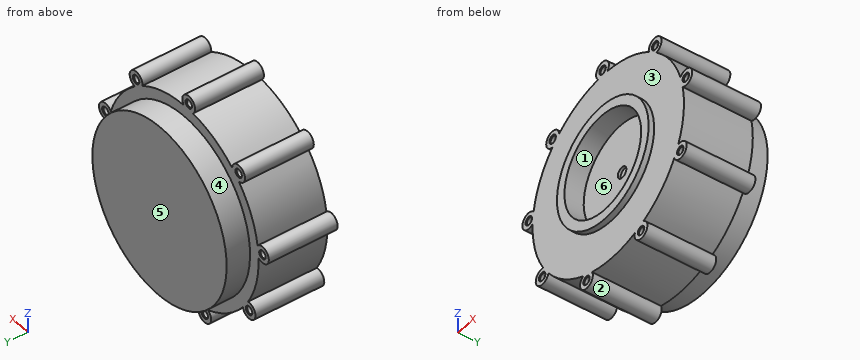
```python
from build123d import *

# Parameters (mm, degrees)
SKETCH_1_R                   = 3
SKETCH_1_R_2                 = 35.5
EXTRUDE_1_DEPTH              = 25
HOLE_WIZARD_M3_1_D           = 2.5
HOLE_WIZARD_M3_1_DEPTH       = 8
HOLE_WIZARD_M3_1_CSINK_D     = 3.05
HOLE_WIZARD_M3_1_CSINK_ANGLE = 90
HOLE_WIZARD_M3_1_TIP         = 0.751075774
SKETCH_7_R                   = 21.5
SKETCH_7_R_2                 = 18
EXTRUDE_3_DEPTH              = 2
CUT_EXTRUDE_START            = -5
SKETCH_8_R                   = 18
CUT_EXTRUDE_2_DEPTH          = 5
SKETCH_9_R                   = 2
CUT_EXTRUDE_3_DEPTH          = 1
SKETCH_11_R                  = 31.5
EXTRUDE_4_DEPTH              = 8.5
HOLE_WIZARD_M3_4_D           = 2.5
HOLE_WIZARD_M3_4_DEPTH       = 8
HOLE_WIZARD_M3_4_CSINK_D     = 3.05
HOLE_WIZARD_M3_4_CSINK_ANGLE = 90
HOLE_WIZARD_M3_4_TIP         = 0.751075774


with BuildPart() as part:
    # 草图1 → 凸台-拉伸1 (new body)
    with BuildSketch(Plane(origin=(0, 0, 0), x_dir=(1, 0, 0), z_dir=(0, 1, 0))):
        with Locations((-31.034181612, 21.050643022)):
            Circle(SKETCH_1_R)
        Circle(SKETCH_1_R_2)
        with Locations((-37.304654882, -3.822659306)):
            Circle(SKETCH_1_R)
        with Locations((-26.119865536, -26.907296861)):
            Circle(SKETCH_1_R)
        with Locations((-2.713300817, -37.401711173)):
            Circle(SKETCH_1_R)
        with Locations((21.96284751, -30.395449154)):
            Circle(SKETCH_1_R)
        with Locations((36.362335397, -9.166818668)):
            Circle(SKETCH_1_R)
        with Locations((33.747482429, 16.351068151)):
            Circle(SKETCH_1_R)
        with Locations((15.341807372, 34.21810846)):
            Circle(SKETCH_1_R)
        with Locations((-10.24246986, 36.074115528)):
            Circle(SKETCH_1_R)
        Circle(SKETCH_1_R_2)
        with Locations((-37.304654882, -3.822659306)):
            Circle(SKETCH_1_R)
        Circle(SKETCH_1_R_2)
        with Locations((-37.304654882, -3.822659306)):
            Circle(SKETCH_1_R)
        Circle(SKETCH_1_R_2)
        with Locations((-26.119865536, -26.907296861)):
            Circle(SKETCH_1_R)
        Circle(SKETCH_1_R_2)
        with Locations((-26.119865536, -26.907296861)):
            Circle(SKETCH_1_R)
        Circle(SKETCH_1_R_2)
        with Locations((-2.713300817, -37.401711173)):
            Circle(SKETCH_1_R)
        Circle(SKETCH_1_R_2)
        with Locations((-2.713300817, -37.401711173)):
            Circle(SKETCH_1_R)
        Circle(SKETCH_1_R_2)
        with Locations((21.96284751, -30.395449154)):
            Circle(SKETCH_1_R)
        Circle(SKETCH_1_R_2)
        with Locations((21.96284751, -30.395449154)):
            Circle(SKETCH_1_R)
        Circle(SKETCH_1_R_2)
        with Locations((36.362335397, -9.166818668)):
            Circle(SKETCH_1_R)
        Circle(SKETCH_1_R_2)
        with Locations((36.362335397, -9.166818668)):
            Circle(SKETCH_1_R)
        Circle(SKETCH_1_R_2)
        with Locations((33.747482429, 16.351068151)):
            Circle(SKETCH_1_R)
        Circle(SKETCH_1_R_2)
        with Locations((33.747482429, 16.351068151)):
            Circle(SKETCH_1_R)
        Circle(SKETCH_1_R_2)
        with Locations((15.341807372, 34.21810846)):
            Circle(SKETCH_1_R)
        Circle(SKETCH_1_R_2)
        with Locations((15.341807372, 34.21810846)):
            Circle(SKETCH_1_R)
        Circle(SKETCH_1_R_2)
        with Locations((-10.24246986, 36.074115528)):
            Circle(SKETCH_1_R)
        Circle(SKETCH_1_R_2)
        with Locations((-10.24246986, 36.074115528)):
            Circle(SKETCH_1_R)
        Circle(SKETCH_1_R_2)
        with Locations((-31.034181612, 21.050643022)):
            Circle(SKETCH_1_R)
        Circle(SKETCH_1_R_2)
        with Locations((-31.034181612, 21.050643022)):
            Circle(SKETCH_1_R)
    extrude(amount=EXTRUDE_1_DEPTH)

    # M3 螺纹孔1
    with Locations(Plane(origin=(-26.119865536, 0, 26.907296861), x_dir=(0, 0, -1), z_dir=(0, -1, 0))):
        with Locations((0, 0), (-10.494414312, 23.406564719), (-3.488152293, 48.082713046), (17.740478193, 62.482200933), (43.258365012, 59.867347965), (61.125405321, 41.461672908), (62.981412389, 15.877395676), (47.957939883, -4.914316076), (23.084637555, -11.184789346)):
            CounterSinkHole(HOLE_WIZARD_M3_1_D / 2, HOLE_WIZARD_M3_1_CSINK_D / 2, depth=HOLE_WIZARD_M3_1_DEPTH, counter_sink_angle=HOLE_WIZARD_M3_1_CSINK_ANGLE)
            with Locations((0, 0, -(HOLE_WIZARD_M3_1_DEPTH + HOLE_WIZARD_M3_1_TIP / 2))):  # 118° drill point
                Cone(0, HOLE_WIZARD_M3_1_D / 2, HOLE_WIZARD_M3_1_TIP, mode=Mode.SUBTRACT)

    # 草图7 → 凸台-拉伸3 (add)
    with BuildSketch(Plane.XZ):
        with Locations(Location((0, 0, 0), (0, 0, 90))):
            Circle(SKETCH_7_R)
        with Locations(Location((0, 0, 0), (0, 0, 270))):
            Circle(SKETCH_7_R_2, mode=Mode.SUBTRACT)
    extrude(amount=EXTRUDE_3_DEPTH)

    # 草图8 → 切除-拉伸2 (cut)
    with BuildSketch(Plane.XZ.offset(CUT_EXTRUDE_START)):
        with Locations(Location((0, 0, 0), (0, 0, 270))):
            Circle(SKETCH_8_R)
    extrude(amount=CUT_EXTRUDE_2_DEPTH, mode=Mode.SUBTRACT)

    # 草图9 → 切除-拉伸3 (cut)
    with BuildSketch(Plane.XZ.offset(-5)):
        with Locations(Location((0, 0, 0), (0, 0, 270))):
            Circle(SKETCH_9_R)
    extrude(amount=-CUT_EXTRUDE_3_DEPTH, mode=Mode.SUBTRACT)

    # 草图11 → 凸台-拉伸4 (add)
    with BuildSketch(Plane(origin=(0, 25, 0), x_dir=(1, 0, 0), z_dir=(0, 1, 0))):
        with Locations(Location((0, 0, 0), (0, 0, 270))):
            Circle(SKETCH_11_R)
    extrude(amount=EXTRUDE_4_DEPTH)

    # M3 螺纹孔4
    with Locations(Plane(origin=(0, 25, 0), x_dir=(1, 0, 0), z_dir=(0, 1, 0))):
        with Locations((-31.034181612, 21.050643022), (-37.304654882, -3.822659306), (-26.119865536, -26.907296861), (-2.713300817, -37.401711173), (21.96284751, -30.395449154), (36.362335397, -9.166818668), (33.747482429, 16.351068151), (15.341807372, 34.21810846), (-10.24246986, 36.074115528)):
            CounterSinkHole(HOLE_WIZARD_M3_4_D / 2, HOLE_WIZARD_M3_4_CSINK_D / 2, depth=HOLE_WIZARD_M3_4_DEPTH, counter_sink_angle=HOLE_WIZARD_M3_4_CSINK_ANGLE)
            with Locations((0, 0, -(HOLE_WIZARD_M3_4_DEPTH + HOLE_WIZARD_M3_4_TIP / 2))):  # 118° drill point
                Cone(0, HOLE_WIZARD_M3_4_D / 2, HOLE_WIZARD_M3_4_TIP, mode=Mode.SUBTRACT)


solid = part.part
```
Could you check a few things on this model? Use its own coordinates, in mm. Face numbers are marked on the shaded views. A direction names the side the tool comes from. Give positions to 0.01 mm unless a question says otherwise; leave off trailing zeros. Write each loop counter-clockwise with the first axis right and the second up, starting at its lowest first coordinate (ties: lowest second). Pieces come first, ordered by that corner, then holes. Notation, with made-up numbers: (6, -10) -> (25, -10) arc R25 cw to (25, 11) -> close; hole circle Ø3 at (33.25, 48.5). An arc over 180 degrees is marked (long way). Write each question's results on one line, items separated by ' | '.
1. If we mould it in two halves opening along X, with no side actions, what happens to the marked faces 1, 2, 3 and 4? For each: released by +X, released by -X, zero draft, split by the parting line, or undercut.
Check sheet entries:
face 1: undercut | face 2: undercut | face 3: zero draft | face 4: split by the parting line
2. On a 3-axis mill with a long thin cutter (end or side, diameter ignored), from which of +Z, -Z, +X, -X, +Y, -Y can I reach the whole of each face in a straight line? I mean the marked faces 5 and 6. Say none if no direction works.
Check sheet entries:
face 5: +Z, -Z, +X, -X, +Y | face 6: -Y
3. I want a section at B-B, the plane x = -15. Write out the boundary of the cut face in (y, z).
Check sheet entries:
outline: (-2, -15.4) -> (0, -15.4) -> (0, -32.18) -> (25, -32.18) -> (25, -27.7) -> (33.5, -27.7) -> (33.5, 27.7) -> (25, 27.7) -> (25, 32.18) -> (0, 32.18) -> (0, 15.4) -> (-2, 15.4) -> (-2, 9.95) -> (5, 9.95) -> (5, -9.95) -> (-2, -9.95) -> close
4. I need wall thicknesses on L1, parallel to Y at x = 16, z = -27; L2, parallel to X at y = 6, z = 31; L3, parallel to Z at x = -26, y = 24. Which ranges of each line are inside material? Lowest first, please.
Check sheet entries:
L1: y = 0 to 33.5 | L2: x = -17.3 to 17.3, 19.02 to 20.87, 23.06 to 24.9 | L3: z = -24.17 to 25.66, 28.15 to 29.9
5. Will these pins go through, and if not, where does the flat tip stop? pin 1 Ø2 at (x, z) = (33.75, -16.35) entering from -Y; pin 2 Ø2 at (x, z) = (-37.3, 3.82) entering from +Y; pin 3 Ø5 at (y, z) = (3, 0.5) entering from -X.
Check sheet entries:
pin 1: stops at y = 8.15 | pin 2: stops at y = 16.85 | pin 3: stops at x = -40.19
6. I want a section at A-A, the plane y = 26.5. Write out the boundary of the cut face in (x, z).
Check sheet entries:
outline: circle Ø63 at (0, 0)
